from build123d import *

# Parameters (mm, degrees)
F0_R     = 3
F0_R_2   = 2
F1_DEPTH = 50
F2_DEPTH = 60
F3_DEPTH = 60
F4_DEPTH = 70
F5_DEPTH = 70
F6_DEPTH = 70
F8_DEPTH = 2
F9_R     = 5


with BuildPart() as f1:
    # F0 (on Top) → F1 (new body)
    with BuildSketch(Plane.XY):
        Circle(F0_R)
        Circle(F0_R_2, mode=Mode.SUBTRACT)
    extrude(amount=F1_DEPTH)



with BuildPart() as f2:
    # F0 (on Top) → F2 (new body)
    with BuildSketch(Plane.XY):
        with Locations((-8.660254, -15)):
            Circle(F0_R)
        with Locations((-8.660254, -15)):
            Circle(F0_R_2, mode=Mode.SUBTRACT)
    extrude(amount=F2_DEPTH)


with BuildPart() as f3:
    # F0 (on Top) → F3 (new body)
    with BuildSketch(Plane.XY):
        with Locations((8.660254, -15)):
            Circle(F0_R)
        with Locations((8.660254, -15)):
            Circle(F0_R_2, mode=Mode.SUBTRACT)
    extrude(amount=F3_DEPTH)


with BuildPart() as f4:
    # F0 (on Top) → F4 (new body)
    with BuildSketch(Plane.XY):
        with Locations((17.320508, -30)):
            Circle(F0_R)
        with Locations((17.320508, -30)):
            Circle(F0_R_2, mode=Mode.SUBTRACT)
    extrude(amount=F4_DEPTH)


with BuildPart() as f5:
    # F0 (on Top) → F5 (new body)
    with BuildSketch(Plane.XY):
        with Locations((0, -30)):
            Circle(F0_R)
        with Locations((0, -30)):
            Circle(F0_R_2, mode=Mode.SUBTRACT)
    extrude(amount=F5_DEPTH)


with BuildPart() as f6:
    # F0 (on Top) → F6 (new body)
    with BuildSketch(Plane.XY):
        with Locations((-17.320508, -30)):
            Circle(F0_R)
        with Locations((-17.320508, -30)):
            Circle(F0_R_2, mode=Mode.SUBTRACT)
    extrude(amount=F6_DEPTH)


with BuildPart() as f1_1:
    add(f1.part)

    add(f2.part)  # F8 merges F2

    add(f3.part)  # F8 merges F3

    add(f4.part)  # F8 merges F4

    add(f5.part)  # F8 merges F5

    add(f6.part)  # F8 merges F6
    # F7 (on Top) → F8 (join)
    with BuildSketch(Plane.XY):
        Polygon((0, 10), (-25.980762, -35), (25.980762, -35), align=None)
    extrude(amount=F8_DEPTH)

    # F9
    f9_edges = [f1_1.edges().sort_by_distance(p)[0] for p in [
        (0, 10, 1),
        (-25.980762, -35, 1),
        (25.980762, -35, 1),
    ]]
    fillet(f9_edges, radius=F9_R)


solid = f1_1.part
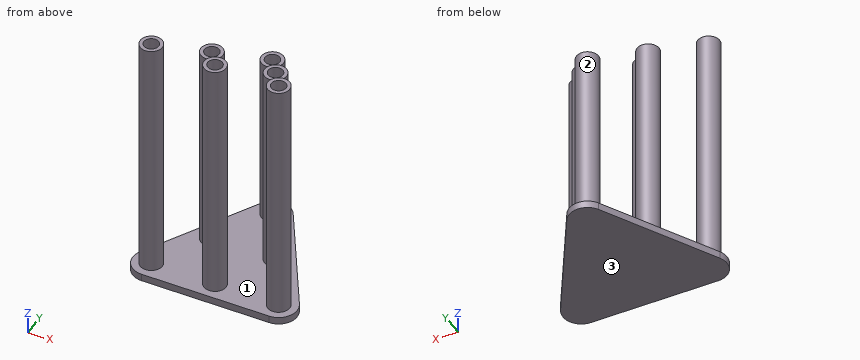
For this review, take the finished solid that the model builds, in its own axes (mm). Face numbers are marked on the shaded views. Coordinates: 2 decimals unless noted, no trailing zeros. Order: outer loops, then holes, each group sorted by start corner. A loop starts at its lowest first (then second) coordinate and runs counter-clockwise, first axis right, second up. Notation, with made-up numbers: (-27, 3.25) - (5, 3.25) arc R29 ccw to (5, 29.25) - close; hole circle Ø5 at (-19.75, -25). An arc over 180 degrees is marked (long way). Use one line per item in the form item = value.
Q1. Consider section D-D (x = 0). Give the boundary of the cut face in (y, z).
Checked values:
outline = (-35, 0) - (5, 0) - (5, 2) - (3, 2) - (3, 50) - (2, 50) - (2, 2) - (-2, 2) - (-2, 50) - (-3, 50) - (-3, 2) - (-27, 2) - (-27, 70) - (-28, 70) - (-28, 2) - (-32, 2) - (-32, 70) - (-33, 70) - (-33, 2) - (-35, 2) - close
Q2. Consider section C-C (y = 0). Give the boundary of the cut face in (x, z).
Checked values:
outline = (-5.77, 0) - (5.77, 0) - (5.77, 2) - (3, 2) - (3, 50) - (2, 50) - (2, 2) - (-2, 2) - (-2, 50) - (-3, 50) - (-3, 2) - (-5.77, 2) - close
Q3. For probe 1 along X at (y, z) = (-30, 21); probe 2 along Y at (x, z) = (0, 27); probe 3 along Y at (x, z) = (-8.5, 32), list the stretches that pass through material, from the lowest coordinate up. Write a range as from..to.
Checked values:
probe_1 = -20.32..-19.32, -15.32..-14.32, -3..-2, 2..3, 14.32..15.32, 19.32..20.32
probe_2 = -33..-32, -28..-27, -3..-2, 2..3
probe_3 = -18..-16.99, -13.01..-12
Q4. For P1, Ø2, axis at x = 17, y = -30, coming from the +Z side; P2, Ø3, axis at x = 8, y = -16, coming from the +Z side; P3, Ø3.5, axis at x = -17.32, y = -30, coming from the -Z side; P4, Ø1, axis at x = 11, z = 46, coming from the -Y side, all flat-tipped, find the tip position at first contact; note any pin that passes through.
Checked values:
P1 = 2
P2 = 60
P3 = 0
P4 = -17.37
Q5. Consider section A-A (z = 43). Give the number of separate pieces and of enclosed holes in the cut face, then the cut area to 3 significant figures.
Checked values:
separate_pieces = 6
enclosed_holes = 6
area = 94.2 mm2
Q6. Draft analysis for pull direction X (two halves, no side actions). For the marked faces 1, 2 and 3, state which applies: +X half, -X half, draft (parallel to the pull), parting line (faces both ways), or undercut.
Checked values:
face_1 = undercut
face_2 = parting line
face_3 = draft
